from build123d import *

# Parameters (mm, degrees)
F0_W     = 121
F0_H     = 57
F1_DEPTH = 54
F3_DEPTH = 57.001
F4_R     = 7
F5_DEPTH = 54.001
F7_DEPTH = 38


with BuildPart() as f1:
    # F0 (on Front) → F1 (new body)
    with BuildSketch(Plane.XZ):
        with Locations((60.5, 28.5)):
            Rectangle(F0_W, F0_H)
    extrude(amount=F1_DEPTH)

    # F2 (on face) → F3 (cut, through all)
    with BuildSketch(Plane.XY.offset(57)):
        Polygon((121, -22), (22, -54), (121, -54), align=None)
    extrude(amount=-F3_DEPTH, mode=Mode.SUBTRACT)

    # F4 (on Front) → F5 (cut, through all)
    with BuildSketch(Plane.XZ):
        with Locations((44, 41)):
            Circle(F4_R)
        with Locations((77, 12)):
            Circle(F4_R)
    extrude(amount=F5_DEPTH, mode=Mode.SUBTRACT)

    # F6 (on face) → F7 (cut)
    with BuildSketch(Plane.XZ.offset(54)):
        Polygon((59, 0), (121, 0), (121, 11), (62, 57), (0, 57), (0, 46), align=None)
    extrude(amount=-F7_DEPTH, mode=Mode.SUBTRACT)


solid = f1.part
Work out the finished part from the listing and answer in its coordinate system (mm). A direction names the side the tool comes from. Coordinates: 2 decimals unless noted, no trailing zeros. Order: outer loops, then holes, each group sorted by start corner. A loop starts at its lowest first (then second) coordinate and runs counter-clockwise, first axis right, second up. Notation, with made-up numbers: (34.5, 60) - (43.5, 60) arc R11 ccw to (43.5, 73) - close; hole circle Ø4 at (64.5, 82.5). An arc over 180 degrees is marked (long way). Put each result on its own line as item: value. Start each with the question number.
1) Find section D-D (y = -31). Give the vertices of the cut face in (x, z).
2) Find the intervals of material crossed by line 1 (X direction, y = -9.5, z = 12); line 2 (X direction, y = -6, z = 41); line 3 (Z direction, x = 77, y = -5.5), in increasing order. Write a range as from..to.
3) Find section B-B (z = 13.5). Give the vertices of the cut face in (x, y).
4) Find section A-A (x = 77). Give the vertices of the cut face in (y, z).
5) A flat-ended cylindrical pin translates along its axis: pin 1 (17 mm diameter, centred on x = 49.5, z = 19, fed in from -Y). Find the tip coordinate at first contact, or state that the pin passes through.
6) For faces 4 (the flat face through (11, -54, 18)), 5 (the flat face through (60, -16, 29)), 6 (the flat face through (85.357, -25.925, 38.789)), 7 (the flat face through (29.09, -35.27, 23.32)), 8 (the cylindrical face through (47.763, -7.888, 46.902)), determine the directions among +Z, -Z, +X, -X, +Y, -Y from which every point of the face is accessible in a straight line to the end or side of a thin tool.
7) Find section C-C (y = -6). Give the vertices of the cut face in (x, z), plus the area to 3 significant figures.
8) For a pull along X with two mould halves and no side action, classify faces 1 (the cylindrical face through (71.445, -7.888, 7.741)), 2 (the flat face through (32.537, -50.594, 8.215)), 3 (the flat face through (60, -11, 57)) as released by +X, released by -X, zero draft, split by the parting line, or undercut.
Results list:
1. outline: (0, 0) - (59, 0) - (0, 46) - close; (62, 57) - (93.16, 32.71) - (93.16, 57) - close
2. line 1: x = 0..70, 84..121
2. line 2: x = 0..37, 51..121
2. line 3: z = 0..5, 19..57
3. outline: (0, -54) - (22, -54) - (41.68, -47.64) - (41.68, -16) - (70.16, -16) - (70.16, 0) - (0, 0) - close; (83.84, -16) - (117.79, -16) - (117.79, -23.04) - (121, -22) - (121, 0) - (83.84, 0) - close
4. outline: (-36.22, 45.31) - (-16, 45.31) - (-16, 19) - (0, 19) - (0, 57) - (-36.22, 57) - close; (-16, 0) - (0, 0) - (0, 5) - (-16, 5) - close
5. pin 1: stops at y = -16
6. face 4: +Z, -Z, +X, -X, -Y
6. face 5: -Y
6. face 6: -Z, -Y
6. face 7: +Z, -Y
6. face 8: +Y, -Y
7. outline: (0, 0) - (121, 0) - (121, 57) - (0, 57) - close; hole circle Ø14 at (44, 41); hole circle Ø14 at (77, 12)
7. area: 6,590 mm^2
8. face 1: undercut
8. face 2: released by +X
8. face 3: zero draft
